Verification items for the finished model (mm, model axes). Face numbers are marked on the shaded views. A direction names the side the tool comes from. Round coordinates to 2 decimals unless told otherwise and drop trailing zeros. Order: outer loops, then holes, each group sorted by start corner. A loop starts at its lowest first (then second) coordinate and runs counter-clockwise, first axis right, second up. Notation, with made-up numbers: (-11.75, -15.75) -> (-6.75, -15.75) arc R17 cw to (-6.75, -5.75) -> close; hole circle Ø7 at (57, -32). An arc over 180 degrees is marked (long way). Write item = value, one per line. Start each with the question number.
from build123d import *

# Parameters (mm, degrees)
BOSS_EXTRUDE1_DEPTH      = 40
CUT_EXTRUDE1_START       = -37
CUT_EXTRUDE1_DEPTH       = 37
M2_CLEARANCE_HOLE1_D     = 2.4
M2_CLEARANCE_HOLE1_DEPTH = 15
M2_CLEARANCE_HOLE1_TIP   = 0.721032743
SKETCH7_R                = 2.5
CUT_EXTRUDE2_DEPTH       = 7


with BuildPart() as part:
    # Sketch1 → Boss-Extrude1 (new body)
    with BuildSketch(Plane(origin=(0, 0, 0), x_dir=(1, 0, 0), z_dir=(0, 1, 0))):
        with BuildLine():
            Line((-115, 25), (115, 25))
            ThreePointArc((115, 25), (118.535533906, 23.535533906), (120, 20))
            Line((120, 20), (120, -20))
            ThreePointArc((120, -20), (118.535533906, -23.535533906), (115, -25))
            Line((115, -25), (-115, -25))
            ThreePointArc((-115, -25), (-118.535533906, -23.535533906), (-120, -20))
            Line((-120, -20), (-120, 20))
            ThreePointArc((-120, 20), (-118.535533906, 23.535533906), (-115, 25))
        make_face()
    extrude(amount=BOSS_EXTRUDE1_DEPTH)

    # Sketch2 → Cut-Extrude1 (cut)
    with BuildSketch(Plane(origin=(0, 40, 0), x_dir=(1, 0, 0), z_dir=(0, 1, 0)).offset(CUT_EXTRUDE1_START)):
        with BuildLine():
            ThreePointArc((110.189543071, 21.363636364), (111.464466094, 16.464466094), (116.363636364, 15.189543071))
            ThreePointArc((116.363636364, 15.189543071), (116.801511345, 15.107359395), (117, 14.708497378))
            Line((117, 14.708497378), (117, -14.708497378))
            ThreePointArc((117, -14.708497378), (116.801511345, -15.107359395), (116.363636364, -15.189543071))
            ThreePointArc((116.363636364, -15.189543071), (111.464466094, -16.464466094), (110.189543071, -21.363636364))
            ThreePointArc((110.189543071, -21.363636364), (110.107359395, -21.801511345), (109.708497378, -22))
            Line((109.708497378, -22), (-109.708497378, -22))
            ThreePointArc((-109.708497378, -22), (-110.107359395, -21.801511345), (-110.189543071, -21.363636364))
            ThreePointArc((-110.189543071, -21.363636364), (-111.464466094, -16.464466094), (-116.363636364, -15.189543071))
            ThreePointArc((-116.363636364, -15.189543071), (-116.801511345, -15.107359395), (-117, -14.708497378))
            Line((-117, -14.708497378), (-117, 14.708497378))
            ThreePointArc((-117, 14.708497378), (-116.801511345, 15.107359395), (-116.363636364, 15.189543071))
            ThreePointArc((-116.363636364, 15.189543071), (-111.464466094, 16.464466094), (-110.189543071, 21.363636364))
            ThreePointArc((-110.189543071, 21.363636364), (-110.107359395, 21.801511345), (-109.708497378, 22))
            Line((-109.708497378, 22), (109.708497378, 22))
            ThreePointArc((109.708497378, 22), (110.107359395, 21.801511345), (110.189543071, 21.363636364))
        make_face()
    extrude(amount=CUT_EXTRUDE1_DEPTH, mode=Mode.SUBTRACT)

    # M2 Clearance Hole1
    with Locations(Plane(origin=(-115, 40, -20), x_dir=(0, 0, 1), z_dir=(0, 1, 0))):
        with Locations((0, 0), (40, 0), (40, 230), (0, 230)):
            Hole(M2_CLEARANCE_HOLE1_D / 2, depth=M2_CLEARANCE_HOLE1_DEPTH)
            with Locations((0, 0, -(M2_CLEARANCE_HOLE1_DEPTH + M2_CLEARANCE_HOLE1_TIP / 2))):  # 118° drill point
                Cone(0, M2_CLEARANCE_HOLE1_D / 2, M2_CLEARANCE_HOLE1_TIP, mode=Mode.SUBTRACT)

    # Sketch7 → Cut-Extrude2 (cut)
    with BuildSketch(Plane(origin=(120, 0, 0), x_dir=(0, 0, -1), z_dir=(1, 0, 0))):
        with Locations((0, 19.817767005)):
            Circle(SKETCH7_R)
    extrude(amount=-CUT_EXTRUDE2_DEPTH, mode=Mode.SUBTRACT)


solid = part.part
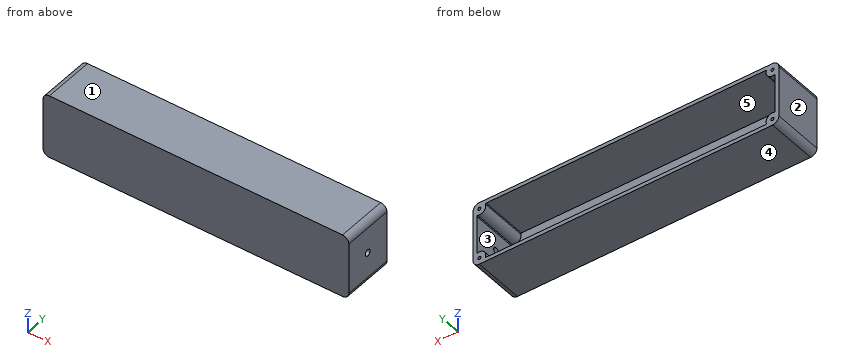
(1) Scan lines: line 1 along X through (y, z) = (34, 20); line 2 along Z through (x, y) = (115, 29); line 3 along X through (y, z) = (25.5, -1). Record each from-to range of solid material in increasing order. Write a range as from..to.
(2) Cross-section at A-A (z = 0). Enter the section's corners in (x, y), and give its area (3 significant figures).
(3) Cross-section at D-D (y = 14). Enter the section's corners in (x, z).
(4) Depth check by flat-ended pin: pin 1 (2 mm diameter, centred on x = -115, z = -20, fed in from +Y); pin 2 (6 mm diameter, centred on x = 88.5, z = -6, fed in from +Y). Enter the tip coordinate at first touch or a pass-through.
(5) Draft check along X on the marked faces 1, 2 and 3. Enter one of: +X half, -X half, draft (parallel to the pull), parting line (faces both ways), or undercut.
(6) Cross-section at B-B (x = -80). Enter the section's corners in (y, z).
(7) Set-up check for the marked faces 4 and 5: record each of +Z, -Z, +X, -X, +Y, -Y from which the full face is reachable in a straight line by a thin tool's end or side.
(8) Cross-section at C-C (y = 36). Enter the section's corners in (x, z).
Outcome:
q1.line_1 = -120..-116.2, -113.8..-110, 110..113.8, 116.2..120
q1.line_2 = -25..-21.2, -18.8..-15, 15..18.8, 21.2..25
q1.line_3 = -120..-117, 117..120
q2.outline = (-120, 0) -> (120, 0) -> (120, 17.32) -> (117, 17.32) -> (117, 3) -> (-117, 3) -> (-117, 40) -> (-120, 40) -> close; (117, 22.32) -> (120, 22.32) -> (120, 40) -> (117, 40) -> close
q2.area = 927 mm^2
q3.outline = (-120, -20) arc R5 ccw to (-115, -25) -> (115, -25) arc R5 ccw to (120, -20) -> (120, 20) arc R5 ccw to (115, 25) -> (-115, 25) arc R5 ccw to (-120, 20) -> close; hole (-117, -14.71) arc R0.5 ccw to (-116.36, -15.19) arc R5 cw to (-110.19, -21.36) arc R0.5 ccw to (-109.71, -22) -> (109.71, -22) arc R0.5 ccw to (110.19, -21.36) arc R5 cw to (116.36, -15.19) arc R0.5 ccw to (117, -14.71) -> (117, 14.71) arc R0.5 ccw to (116.36, 15.19) arc R5 cw to (110.19, 21.36) arc R0.5 ccw to (109.71, 22) -> (-109.71, 22) arc R0.5 ccw to (-110.19, 21.36) arc R5 cw to (-116.36, 15.19) arc R0.5 ccw to (-117, 14.71) -> close
q4.pin_1 = 24.88
q4.pin_2 = 3
q5.face_1 = draft
q5.face_2 = -X half
q5.face_3 = undercut
q6.outline = (0, -25) -> (40, -25) -> (40, -22) -> (3, -22) -> (3, 22) -> (40, 22) -> (40, 25) -> (0, 25) -> close
q7.face_4 = -Z, +X, -X, +Y, -Y
q7.face_5 = +Y
q8.outline = (-120, -20) arc R5 ccw to (-115, -25) -> (115, -25) arc R5 ccw to (120, -20) -> (120, 20) arc R5 ccw to (115, 25) -> (-115, 25) arc R5 ccw to (-120, 20) -> close; hole (-117, -14.71) arc R0.5 ccw to (-116.36, -15.19) arc R5 cw to (-110.19, -21.36) arc R0.5 ccw to (-109.71, -22) -> (109.71, -22) arc R0.5 ccw to (110.19, -21.36) arc R5 cw to (116.36, -15.19) arc R0.5 ccw to (117, -14.71) -> (117, 14.71) arc R0.5 ccw to (116.36, 15.19) arc R5 cw to (110.19, 21.36) arc R0.5 ccw to (109.71, 22) -> (-109.71, 22) arc R0.5 ccw to (-110.19, 21.36) arc R5 cw to (-116.36, 15.19) arc R0.5 ccw to (-117, 14.71) -> close; hole circle Ø2.4 at (-115, -20); hole circle Ø2.4 at (-115, 20); hole circle Ø2.4 at (115, -20); hole circle Ø2.4 at (115, 20)
